Geometry check sheet. Reference: drawing and pictorial views, mm from the part's lowest x, y, z. A direction names the side the tool comes from. Round coordinates to 2 decimals unless told otherwise and drop trailing zeros. Write each loop counter-clockwise with the first axis right and the second up, starting at its lowest first coordinate (ties: lowest second). Pieces come first, ordered by that corner, then holes. Notation, with made-up numbers: M 70.25,63 L 89.25,63 A28 ccw 89.25,90 Z; hole C 84.5,31.5 d5. An arc over 180 degrees is marked long. One line per item, written item: value. Start each with the question number.
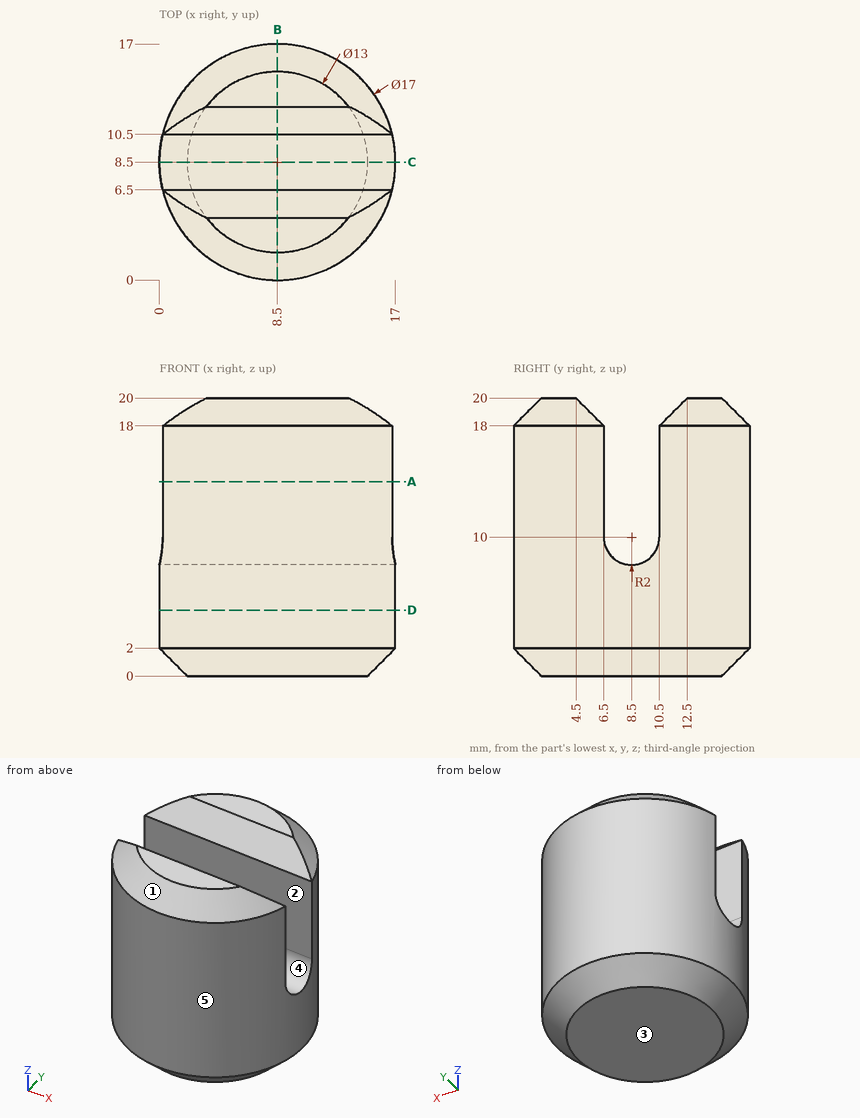
1) Cross-section at C-C (y = 8.5). Record the boundary of the cut face in (x, z).
2) Thickness scan on line 1 (Y direction, x = 1, z = 13); line 2 (Y direction, x = 15, z = 15.5); line 3 (Y direction, x = 3.75, z = 5.5). Record the ranges inside material, lowest first.
3) Cross-section at D-D (z = 4.75). Record the boundary of the cut face in (x, y), then the cut area to 3 significant figures.
4) Mould release check, pull along Y, two halves, no side actions. Record for the marked faces 3, 4 and 5: pulls with the +Y half, pulls with the -Y half, needs draft (parallel to the pull), parting line crosses it, or undercut.
5) Cross-section at B-B (x = 8.5). Record the boundary of the cut face in (y, z), then the cut area to 3 significant figures.
6) Gauge pin test, flat ends, axial feed: pin 1 Ø2.5 at (x, z) = (12, 15) entering from -Y; pin 2 Ø5 at (x, z) = (12, 15.5) entering from -Y; pin 3 Ø1 at (x, y) = (8.5, 9.5) entering from +Z. Record the tip position at first contact, or that the pin passes through.
7) Cross-section at A-A (z = 14). Record the boundary of the cut face in (x, y), then the cut area to 3 significant figures.
8) Access from +Z, -Z, +X, -X, +Y, -Y to the whole of each face (thin tool, end or side, straight path). Record for the marked faces 1 and 2.
Results below:
1. outline: M 0,2 L 2,0 L 15,0 L 17,2 L 17,8 L 0,8 Z
2. line 1: y = 4.5 to 6.5, 10.5 to 12.5
2. line 2: y = 3.02 to 6.5, 10.5 to 13.98
2. line 3: y = 1.45 to 15.55
3. outline: C 8.5,8.5 d17
3. area: 227 mm²
4. face 3: needs draft
4. face 4: undercut
4. face 5: parting line crosses it
5. outline: M 0,2 L 2,0 L 15,0 L 17,2 L 17,18 L 15,20 L 12.5,20 L 10.5,18 L 10.5,10 A2 cw 6.5,10 L 6.5,18 L 4.5,20 L 2,20 L 0,18 Z
5. area: 282 mm²
6. pin 1: stops at y = 0.3
6. pin 2: stops at y = 0.06
6. pin 3: stops at z = 8.68
7. outline: M 0.24,6.5 A8.5 ccw 16.76,6.5 Z; M 0.24,10.5 L 16.76,10.5 A8.5 ccw Z
7. area: 160 mm²
8. face 1: +Z, -Y
8. face 2: +Z, +X, -X
